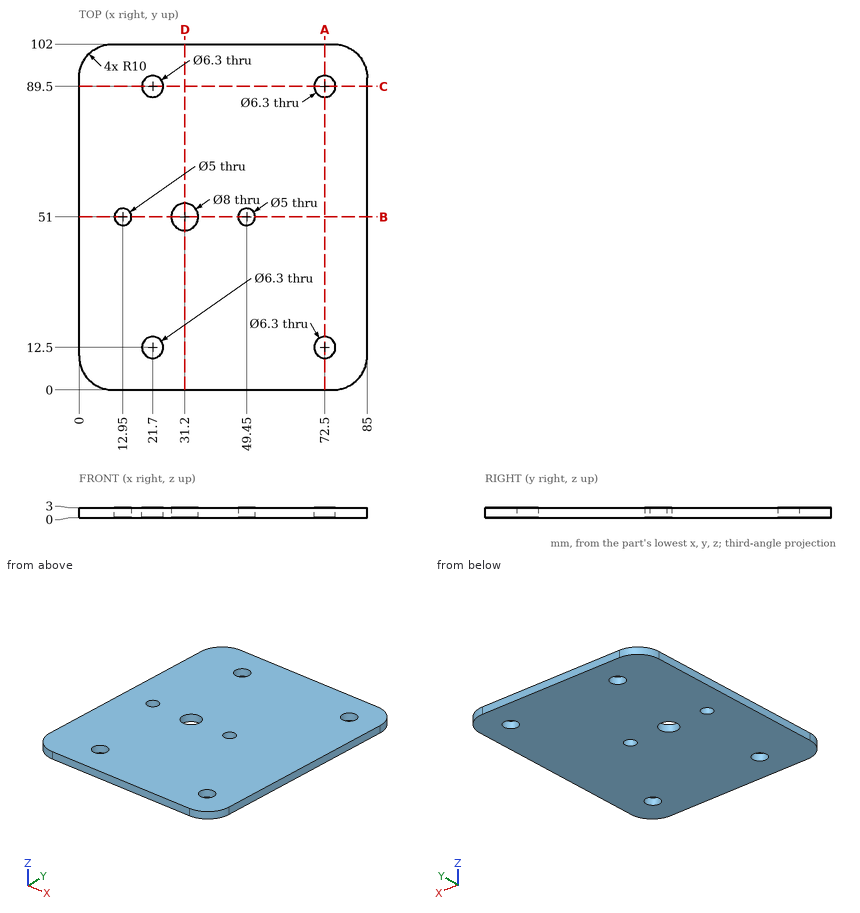
Print and shaded views of the part. All mm, measured from the part's lowest x, y and z. Give positions to 0.01 mm unless a question says otherwise; leave off trailing zeros. Write each loop counter-clockwise with the first axis right and the second up, starting at its lowest first coordinate (ties: lowest second). Pieces come first, ordered by that corner, then holes. Notation, with made-up numbers: (-10.5, 32.5) -> (40.5, 32.5) arc R14 ccw to (40.5, 46.5) -> close; hole circle Ø11 at (-3.75, 49.25). An arc over 180 degrees is marked (long way). Write each question's results on one line, items separated by ' | '.
1. Cut at D-D, the plane x = 31.2. Write the cut outline in (y, z).
Geometry check:
outline: (0, 0) -> (47, 0) -> (47, 3) -> (0, 3) -> close; (55, 0) -> (102, 0) -> (102, 3) -> (55, 3) -> close
2. Cut at A-A, the plane x = 72.5. Write the cut outline in (y, z).
Geometry check:
outline: (0, 0) -> (9.35, 0) -> (9.35, 3) -> (0, 3) -> close; (15.65, 0) -> (86.35, 0) -> (86.35, 3) -> (15.65, 3) -> close; (92.65, 0) -> (102, 0) -> (102, 3) -> (92.65, 3) -> close
3. Drop a flat-ended pin along its axis: P1, Ø4.5, axis at x = 49.45, y = 51, coming from the +Z side. Give the stop position or say it passes through.
Geometry check:
P1: through
4. Cut at B-B, the plane y = 51. Write the cut outline in (x, z).
Geometry check:
outline: (0, 0) -> (10.45, 0) -> (10.45, 3) -> (0, 3) -> close; (15.45, 0) -> (27.2, 0) -> (27.2, 3) -> (15.45, 3) -> close; (35.2, 0) -> (46.95, 0) -> (46.95, 3) -> (35.2, 3) -> close; (51.95, 0) -> (85, 0) -> (85, 3) -> (51.95, 3) -> close
5. Wall check: probe 1 along X at (y, z) = (12.5, 1.35); probe 2 along Y at (x, z) = (72.5, 0.6); probe 3 along Y at (x, z) = (24, 1.5). Give the ranges that are in metal, low to high. Write a range as [from, to].
Geometry check:
probe 1: [0, 18.55], [24.85, 69.35], [75.65, 85] | probe 2: [0, 9.35], [15.65, 86.35], [92.65, 102] | probe 3: [0, 10.35], [14.65, 87.35], [91.65, 102]
6. Cut at C-C, the plane y = 89.5. Write the cut outline in (x, z), then the cut area to 3 significant figures.
Geometry check:
outline: (0, 0) -> (18.55, 0) -> (18.55, 3) -> (0, 3) -> close; (24.85, 0) -> (69.35, 0) -> (69.35, 3) -> (24.85, 3) -> close; (75.65, 0) -> (85, 0) -> (85, 3) -> (75.65, 3) -> close | area: 217 mm²
